Could you check a few things on this model? Use its own coordinates, in mm. Round coordinates to 2 decimals unless told otherwise and drop trailing zeros. Write each loop counter-clockwise with the first axis right and the second up, starting at its lowest first coordinate (ties: lowest second). Pieces come first, ordered by that corner, then holes. Notation, with made-up numbers: (-28.75, -12.75) - (7.25, -12.75) arc R6 cw to (7.25, -8.75) - close; hole circle Ø1 at (83.25, -0.75). An arc over 180 degrees is marked (long way). Write each question's results on one line, items separated by ' | '. Start each with the question number.
(1) Thinking about a two-plate mould opening in X: for faces 1 (the flat face through (88, 11.9, 3)), 2 (the cylindrical face through (-124.88, 5.5, 2.96)), 3 (the flat face through (-2, 2, 6)), 4 (the flat face through (54.9, 78, 3)), which applies, +X half, -X half, draft (parallel to the pull), parting line (faces both ways), or undercut?
(2) Imagine slicing it at B-B on y = -96.5. Write out the boundary of the cut face in (x, z), then the cut area to 3 significant figures.
(3) Please list where these lines run through material, in increasing order: line 1 (X direction, y = 20.5, z = 1.95); line 2 (X direction, y = -8, z = 4.85); line 3 (X direction, y = -81, z = 3.2). Write a range as [from, to].
(4) Imagine slicing it at C-C on z = 2.95. State how many separate pieces and enclosed holes the cut face has, then the cut area to 3 significant figures.
(5) Imagine slicing it at D-D on y = 93.5. Write out the boundary of the cut face in (x, z).
(6) Imagine slicing it at A-A on y = 9. Write out the boundary of the cut face in (x, z), then the cut area to 3 significant figures.
(7) For P1, Ø2, axis at x = -37.5, y = -31.31, coming from the +Z side; P2, Ø5, axis at x = 67, y = 78, coming from the -Z side; P3, Ø1.8, axis at x = 100.5, z = 2, coming from the +Y side; P4, Ø1.8, axis at y = 12.5, z = 4.5, coming from the +X side, each with a flat end and sliding along its axis, tell me the tip position at first contact or that it passes through.
```python
from build123d import *

# Parameters (mm, degrees)
ESQUISSE1_R                  = 125
BOSS_EXTRU_1_DEPTH           = 6
ESQUISSE2_W                  = 15
ESQUISSE2_H                  = 76
ENL_V_MAT_EXTRU_1_DEPTH      = 7
ESQUISSE3_R                  = 2
ESQUISSE3_W                  = 8.2
ESQUISSE3_H                  = 6.2
ENL_V_MAT_EXTRU_2_DEPTH      = 7
R_P_TITION_CIRCULAIRE1_COUNT = 4
ESQUISSE4_W                  = 6.2
ESQUISSE4_H                  = 8.2
ENL_V_MAT_EXTRU_3_DEPTH      = 7
ENL_V_MAT_EXTRU_4_REACH      = 8
ESQUISSE8_R                  = 1.65
ESQUISSE8_W                  = 72
ESQUISSE8_H                  = 27
ENL_V_MAT_EXTRU_5_REACH      = 8
ESQUISSE9_R                  = 1.65
ESQUISSE9_R_2                = 1.15
ESQUISSE9_W                  = 12
ESQUISSE9_H                  = 22.7


with BuildPart() as part:
    # Esquisse1 → Boss.-Extru.1 (new body)
    with BuildSketch(Plane.XY):
        Circle(ESQUISSE1_R)
    extrude(amount=BOSS_EXTRU_1_DEPTH)

    # Esquisse2 → Enl_v. mat.-Extru.1 (cut, through all)
    with BuildSketch(Plane.XY.offset(6)):
        with Locations((-102.5, 0)):
            Rectangle(ESQUISSE2_W, ESQUISSE2_H)
    enl_v_mat_extru_1 = extrude(amount=-ENL_V_MAT_EXTRU_1_DEPTH, mode=Mode.SUBTRACT)

    # Sym_trie1: Enl_v. mat.-Extru.1 across plane
    add(enl_v_mat_extru_1.mirror(Plane(origin=(0, 0, 0), x_dir=(0, 0, 1), z_dir=(1, 0, 0))), mode=Mode.SUBTRACT)

    # Esquisse3 → Enl_v. mat.-Extru.2 (cut, through all)
    with BuildSketch(Plane(origin=(0, 0, 0), x_dir=(-1, 0, 0), z_dir=(0, 0, -1))):
        with Locations((-67, 78)):
            Circle(ESQUISSE3_R)
        with Locations((-75, 78)):
            Rectangle(ESQUISSE3_W, ESQUISSE3_H)
        with Locations((-59, 78)):
            Rectangle(ESQUISSE3_W, ESQUISSE3_H)
    enl_v_mat_extru_2 = extrude(amount=-ENL_V_MAT_EXTRU_2_DEPTH, mode=Mode.SUBTRACT)

    # R_p_tition circulaire1: Enl_v. mat.-Extru.2 ×4 about axis
    r_p_tition_circulaire1_axis = Axis((0, 0, 0), (0, 0, 1))
    for i in range(1, R_P_TITION_CIRCULAIRE1_COUNT):
        add(enl_v_mat_extru_2.rotate(r_p_tition_circulaire1_axis, i * 360 / R_P_TITION_CIRCULAIRE1_COUNT), mode=Mode.SUBTRACT)

    # Esquisse4 → Enl_v. mat.-Extru.3 (cut, through all)
    with BuildSketch(Plane(origin=(0, 0, 0), x_dir=(-1, 0, 0), z_dir=(0, 0, -1))):
        with Locations((88, 16)):
            Rectangle(ESQUISSE4_W, ESQUISSE4_H)
        with Locations((88, -16)):
            Rectangle(ESQUISSE4_W, ESQUISSE4_H)
        with Locations((88, 0)):
            Rectangle(ESQUISSE4_W, ESQUISSE4_H)
    enl_v_mat_extru_3 = extrude(amount=-ENL_V_MAT_EXTRU_3_DEPTH, mode=Mode.SUBTRACT)

    # Sym_trie2: Enl_v. mat.-Extru.3 across plane
    add(enl_v_mat_extru_3.mirror(Plane(origin=(0, 0, 0), x_dir=(0, 0, 1), z_dir=(1, 0, 0))), mode=Mode.SUBTRACT)

    # Esquisse8 → Enl_v. mat.-Extru.4 (cut, up to next)
    with BuildSketch(Plane.XY.offset(6), mode=Mode.PRIVATE) as enl_v_mat_extru_4_sk1:
        with Locations((-37.5, -31.305965203)):
            Circle(ESQUISSE8_R)
    enl_v_mat_extru_4_tool1 = extrude(enl_v_mat_extru_4_sk1.sketch, amount=-ENL_V_MAT_EXTRU_4_REACH, mode=Mode.PRIVATE) & part.part
    add(enl_v_mat_extru_4_tool1.solids().sort_by_distance((-37.5, -31.305965, 6))[0], mode=Mode.SUBTRACT)
    # Esquisse8 → Enl_v. mat.-Extru.4 (cut, up to next)
    with BuildSketch(Plane.XY.offset(6), mode=Mode.PRIVATE) as enl_v_mat_extru_4_sk2:
        with Locations((37.5, -31.305965203)):
            Circle(ESQUISSE8_R)
    enl_v_mat_extru_4_tool2 = extrude(enl_v_mat_extru_4_sk2.sketch, amount=-ENL_V_MAT_EXTRU_4_REACH, mode=Mode.PRIVATE) & part.part
    add(enl_v_mat_extru_4_tool2.solids().sort_by_distance((37.5, -31.305965, 6))[0], mode=Mode.SUBTRACT)
    # Esquisse8 → Enl_v. mat.-Extru.4 (cut, up to next)
    with BuildSketch(Plane.XY.offset(6), mode=Mode.PRIVATE) as enl_v_mat_extru_4_sk3:
        with Locations((37.5, -62.305965203)):
            Circle(ESQUISSE8_R)
    enl_v_mat_extru_4_tool3 = extrude(enl_v_mat_extru_4_sk3.sketch, amount=-ENL_V_MAT_EXTRU_4_REACH, mode=Mode.PRIVATE) & part.part
    add(enl_v_mat_extru_4_tool3.solids().sort_by_distance((37.5, -62.305965, 6))[0], mode=Mode.SUBTRACT)
    # Esquisse8 → Enl_v. mat.-Extru.4 (cut, up to next)
    with BuildSketch(Plane.XY.offset(6), mode=Mode.PRIVATE) as enl_v_mat_extru_4_sk4:
        with Locations((-37.5, -62.305965203)):
            Circle(ESQUISSE8_R)
    enl_v_mat_extru_4_tool4 = extrude(enl_v_mat_extru_4_sk4.sketch, amount=-ENL_V_MAT_EXTRU_4_REACH, mode=Mode.PRIVATE) & part.part
    add(enl_v_mat_extru_4_tool4.solids().sort_by_distance((-37.5, -62.305965, 6))[0], mode=Mode.SUBTRACT)
    # Esquisse8 → Enl_v. mat.-Extru.4 (cut, up to next)
    with BuildSketch(Plane.XY.offset(6), mode=Mode.PRIVATE) as enl_v_mat_extru_4_sk5:
        with Locations((-27.94, -70.967629177)):
            Circle(ESQUISSE8_R)
    enl_v_mat_extru_4_tool5 = extrude(enl_v_mat_extru_4_sk5.sketch, amount=-ENL_V_MAT_EXTRU_4_REACH, mode=Mode.PRIVATE) & part.part
    add(enl_v_mat_extru_4_tool5.solids().sort_by_distance((-27.94, -70.967629, 6))[0], mode=Mode.SUBTRACT)
    # Esquisse8 → Enl_v. mat.-Extru.4 (cut, up to next)
    with BuildSketch(Plane.XY.offset(6), mode=Mode.PRIVATE) as enl_v_mat_extru_4_sk6:
        with Locations((27.94, -70.967629177)):
            Circle(ESQUISSE8_R)
    enl_v_mat_extru_4_tool6 = extrude(enl_v_mat_extru_4_sk6.sketch, amount=-ENL_V_MAT_EXTRU_4_REACH, mode=Mode.PRIVATE) & part.part
    add(enl_v_mat_extru_4_tool6.solids().sort_by_distance((27.94, -70.967629, 6))[0], mode=Mode.SUBTRACT)
    # Esquisse8 → Enl_v. mat.-Extru.4 (cut, up to next)
    with BuildSketch(Plane.XY.offset(6), mode=Mode.PRIVATE) as enl_v_mat_extru_4_sk7:
        with Locations((27.94, -114.147629177)):
            Circle(ESQUISSE8_R)
    enl_v_mat_extru_4_tool7 = extrude(enl_v_mat_extru_4_sk7.sketch, amount=-ENL_V_MAT_EXTRU_4_REACH, mode=Mode.PRIVATE) & part.part
    add(enl_v_mat_extru_4_tool7.solids().sort_by_distance((27.94, -114.147629, 6))[0], mode=Mode.SUBTRACT)
    # Esquisse8 → Enl_v. mat.-Extru.4 (cut, up to next)
    with BuildSketch(Plane.XY.offset(6), mode=Mode.PRIVATE) as enl_v_mat_extru_4_sk8:
        with Locations((-27.94, -114.147629177)):
            Circle(ESQUISSE8_R)
    enl_v_mat_extru_4_tool8 = extrude(enl_v_mat_extru_4_sk8.sketch, amount=-ENL_V_MAT_EXTRU_4_REACH, mode=Mode.PRIVATE) & part.part
    add(enl_v_mat_extru_4_tool8.solids().sort_by_distance((-27.94, -114.147629, 6))[0], mode=Mode.SUBTRACT)
    # Esquisse8 → Enl_v. mat.-Extru.4 (cut, up to next)
    with BuildSketch(Plane.XY.offset(6), mode=Mode.PRIVATE) as enl_v_mat_extru_4_sk9:
        with Locations((0, -46.805965203)):
            Rectangle(ESQUISSE8_W, ESQUISSE8_H)
    enl_v_mat_extru_4_tool9 = extrude(enl_v_mat_extru_4_sk9.sketch, amount=-ENL_V_MAT_EXTRU_4_REACH, mode=Mode.PRIVATE) & part.part
    add(enl_v_mat_extru_4_tool9.solids().sort_by_distance((0, -46.805965, 6))[0], mode=Mode.SUBTRACT)
    # Esquisse8 → Enl_v. mat.-Extru.4 (cut, up to next)
    with BuildSketch(Plane.XY.offset(6), mode=Mode.PRIVATE) as enl_v_mat_extru_4_sk10:
        with BuildLine():
            Line((-22.804705882, -112.497629177), (22.804705882, -112.497629177))
            ThreePointArc((22.804705882, -112.497629177), (24.926026226, -111.618949521), (25.804705882, -109.497629177))
            Line((25.804705882, -109.497629177), (25.804705882, -75.617629177))
            ThreePointArc((25.804705882, -75.617629177), (24.926026226, -73.496308834), (22.804705882, -72.617629177))
            Line((22.804705882, -72.617629177), (-22.804705882, -72.617629177))
            ThreePointArc((-22.804705882, -72.617629177), (-24.926026226, -73.496308834), (-25.804705882, -75.617629177))
            Line((-25.804705882, -75.617629177), (-25.804705882, -109.497629177))
            ThreePointArc((-25.804705882, -109.497629177), (-24.926026226, -111.618949521), (-22.804705882, -112.497629177))
        make_face()
    enl_v_mat_extru_4_tool10 = extrude(enl_v_mat_extru_4_sk10.sketch, amount=-ENL_V_MAT_EXTRU_4_REACH, mode=Mode.PRIVATE) & part.part
    add(enl_v_mat_extru_4_tool10.solids().sort_by_distance((0, -92.557629, 6))[0], mode=Mode.SUBTRACT)

    # Esquisse9 → Enl_v. mat.-Extru.5 (cut, up to next)
    with BuildSketch(Plane.XY.offset(6), mode=Mode.PRIVATE) as enl_v_mat_extru_5_sk1:
        with Locations((-13.75, 62.5)):
            Circle(ESQUISSE9_R)
    enl_v_mat_extru_5_tool1 = extrude(enl_v_mat_extru_5_sk1.sketch, amount=-ENL_V_MAT_EXTRU_5_REACH, mode=Mode.PRIVATE) & part.part
    add(enl_v_mat_extru_5_tool1.solids().sort_by_distance((-13.75, 62.5, 6))[0], mode=Mode.SUBTRACT)
    # Esquisse9 → Enl_v. mat.-Extru.5 (cut, up to next)
    with BuildSketch(Plane.XY.offset(6), mode=Mode.PRIVATE) as enl_v_mat_extru_5_sk2:
        with Locations((13.75, 62.5)):
            Circle(ESQUISSE9_R)
    enl_v_mat_extru_5_tool2 = extrude(enl_v_mat_extru_5_sk2.sketch, amount=-ENL_V_MAT_EXTRU_5_REACH, mode=Mode.PRIVATE) & part.part
    add(enl_v_mat_extru_5_tool2.solids().sort_by_distance((13.75, 62.5, 6))[0], mode=Mode.SUBTRACT)
    # Esquisse9 → Enl_v. mat.-Extru.5 (cut, up to next)
    with BuildSketch(Plane.XY.offset(6), mode=Mode.PRIVATE) as enl_v_mat_extru_5_sk3:
        with Locations((0, 28.75)):
            Circle(ESQUISSE9_R_2)
    enl_v_mat_extru_5_tool3 = extrude(enl_v_mat_extru_5_sk3.sketch, amount=-ENL_V_MAT_EXTRU_5_REACH, mode=Mode.PRIVATE) & part.part
    add(enl_v_mat_extru_5_tool3.solids().sort_by_distance((0, 28.75, 6))[0], mode=Mode.SUBTRACT)
    # Esquisse9 → Enl_v. mat.-Extru.5 (cut, up to next)
    with BuildSketch(Plane.XY.offset(6), mode=Mode.PRIVATE) as enl_v_mat_extru_5_sk4:
        with Locations((0, 1.25)):
            Circle(ESQUISSE9_R_2)
    enl_v_mat_extru_5_tool4 = extrude(enl_v_mat_extru_5_sk4.sketch, amount=-ENL_V_MAT_EXTRU_5_REACH, mode=Mode.PRIVATE) & part.part
    add(enl_v_mat_extru_5_tool4.solids().sort_by_distance((0, 1.25, 6))[0], mode=Mode.SUBTRACT)
    # Esquisse9 → Enl_v. mat.-Extru.5 (cut, up to next)
    with BuildSketch(Plane.XY.offset(6), mode=Mode.PRIVATE) as enl_v_mat_extru_5_sk5:
        with Locations((0, 15)):
            Rectangle(ESQUISSE9_W, ESQUISSE9_H)
    enl_v_mat_extru_5_tool5 = extrude(enl_v_mat_extru_5_sk5.sketch, amount=-ENL_V_MAT_EXTRU_5_REACH, mode=Mode.PRIVATE) & part.part
    add(enl_v_mat_extru_5_tool5.solids().sort_by_distance((0, 15, 6))[0], mode=Mode.SUBTRACT)


solid = part.part
```
Response:
1) face 1: undercut | face 2: parting line | face 3: draft | face 4: undercut
2) outline: (-79.45, 0) - (-25.8, 0) - (-25.8, 6) - (-79.45, 6) - close; (25.8, 0) - (79.45, 0) - (79.45, 6) - (25.8, 6) - close | area: 644 mm²
3) line 1: [-123.31, -110], [-95, -6], [6, 95], [110, 123.31] | line 2: [-124.74, -110], [-95, 95], [110, 124.74] | line 3: [-95.21, -79.1], [-70.9, -63.1], [-54.9, -25.8], [25.8, 95.21]
4) separate pieces: 1 | enclosed holes: 35 | area: 41,700 mm²
5) outline: (-82.96, 0) - (82.96, 0) - (82.96, 6) - (-82.96, 6) - close
6) outline: (-124.68, 0) - (-110, 0) - (-110, 6) - (-124.68, 6) - close; (-95, 0) - (-6, 0) - (-6, 6) - (-95, 6) - close; (6, 0) - (95, 0) - (95, 6) - (6, 6) - close; (110, 0) - (124.68, 0) - (124.68, 6) - (110, 6) - close | area: 1,240 mm²
7) P1: through | P2: z = 0 | P3: y = 75.53 | P4: x = 124.46
